Job drawing, mm, ordinate dimensions from the low corner. One solid piece. A direction names the side the tool comes from. Round coordinates to 2 decimals unless told otherwise and drop trailing zeros. Order: outer loops, then holes, each group sorted by start corner. A loop starts at its lowest first (then second) coordinate and runs counter-clockwise, first axis right, second up. Notation, with made-up numbers: (20.5, 15.25) -> (48.5, 15.25) arc R13 ccw to (48.5, 36.25) -> close; hole circle Ø7 at (17, 41). An arc over 180 degrees is marked (long way). Answer as a JSON object with one key per item and string values. Group by question number.
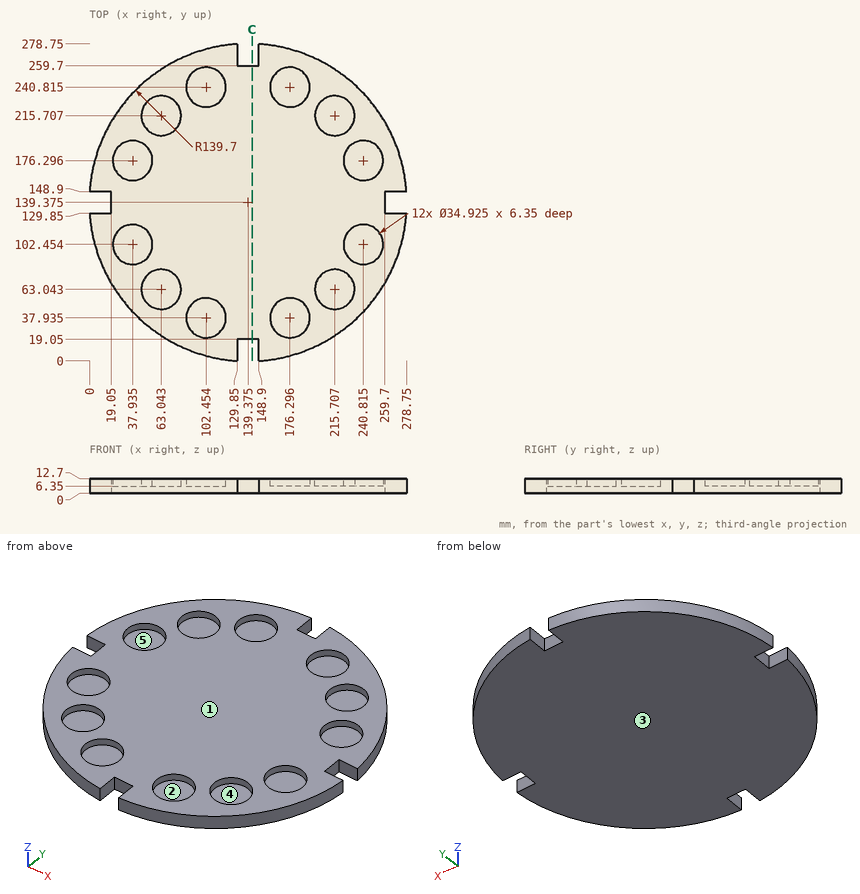
Q1. Drop flat-ended pins along their axis: pin 1 Ø5 at (y, z) = (239.5, 3.5) entering from -X; pin 2 Ø2 at (y, z) = (247.5, 1.5) entering from -X; pin 3 Ø17.5 at (x, y) = (175.5, 30) entering from +Z. Give the stop position or say it passes through.
Q2. Wall check: line 1 (Y direction, x = 100, z = 7.75) (1 decimal); line 2 (Y direction, x = 251, z = 6.5) (1 decimal); line 3 (X direction, y = 251.5, z = 10.75) (1 decimal). Give the ranges that are in metal, low to high. Write a range as [from, to].
Q3. Band-saw the part on C-C (x = 143). List the corners of the cut face in (y, z), plus the area to 3 significant figures.
Q4. Which spindle directions (+Z, -Z, +X, -X, +Y, -Y) get a long thin tool onto all of the face, cutting with end or side? Do the marked faces 1 and 2. Say none if no direction does.
Q5. Two-plate mould, pull along X, no slides. Class the marked faces 3, 4 and 5: +X half, -X half, draft (parallel to the pull), parting line (faces both ways), or undercut.
Completed:
{
 "1": {"pin 1": "x = 39.45", "pin 2": "x = 49.71", "pin 3": "z = 6.35"},
 "2": {"line 1": "[5.3, 20.6], [55.2, 223.5], [258.1, 273.4]", "line 2": "[55.4, 88.3], [116.6, 162.1], [190.5, 223.4]", "line 3": "[56, 88.6], [116.3, 162.5], [190.1, 222.7]"},
 "3": {"outline": "(19.05, 0) -> (259.7, 0) -> (259.7, 12.7) -> (19.05, 12.7) -> close", "area": "3,060 mm2"},
 "4": {"face 1": "+Z, +X, -X, +Y, -Y", "face 2": "+Z"},
 "5": {"face 3": "draft", "face 4": "undercut", "face 5": "undercut"}
}
